The figure shows three views and two pictorial views of one solid part (mm, origin at its lowest corner). Answer the questions. Round coordinates to 2 decimals unless told otherwise and drop trailing zeros. Order: outer loops, then holes, each group sorted by start corner. A loop starts at its lowest first (then second) coordinate and runs counter-clockwise, first axis right, second up. Notation, with made-up numbers: (-4.75, 57) - (1.25, 57) arc R21 ccw to (1.25, 63) - close; hole circle Ø6 at (-28, -29.5). An arc over 180 degrees is marked (long way). Answer as a JSON object with one key per item and string values. Group by question number.
Q1. A cutting plane is placed at A-A on z = 2.25. Determine the outline of the cut face in (x, y).
Q2. A cutting plane is placed at C-C on z = 3.1. Determine the outline of the cut face in (x, y).
Q3. Given pin 1 Ø2 at (x, z) = (3.1, 3.1) entering from +Y, flat-ended and moving along its own axis, determine where the tip first touches the part or whether it passes through.
Q4. A cutting plane is placed at D-D on y = 0.45. Determine the outline of the cut face in (x, z).
Q5. Consider line 1 (Z direction, x = 3.1, y = 0.2); line 2 (X direction, y = 0.55, z = 3.1); line 3 (X direction, y = 0.2, z = 4.25). Determine where each line is inside the solid, lowest interval first.
Q6. A cutting plane is placed at B-B on x = 1.75. Determine the outline of the cut face in (y, z).
Q7. The mould has two halves that part along X. Classify the marked faces 1 and 2: pulls with the +X half, pulls with the -X half, needs draft (parallel to the pull), parting line crosses it, or undercut.
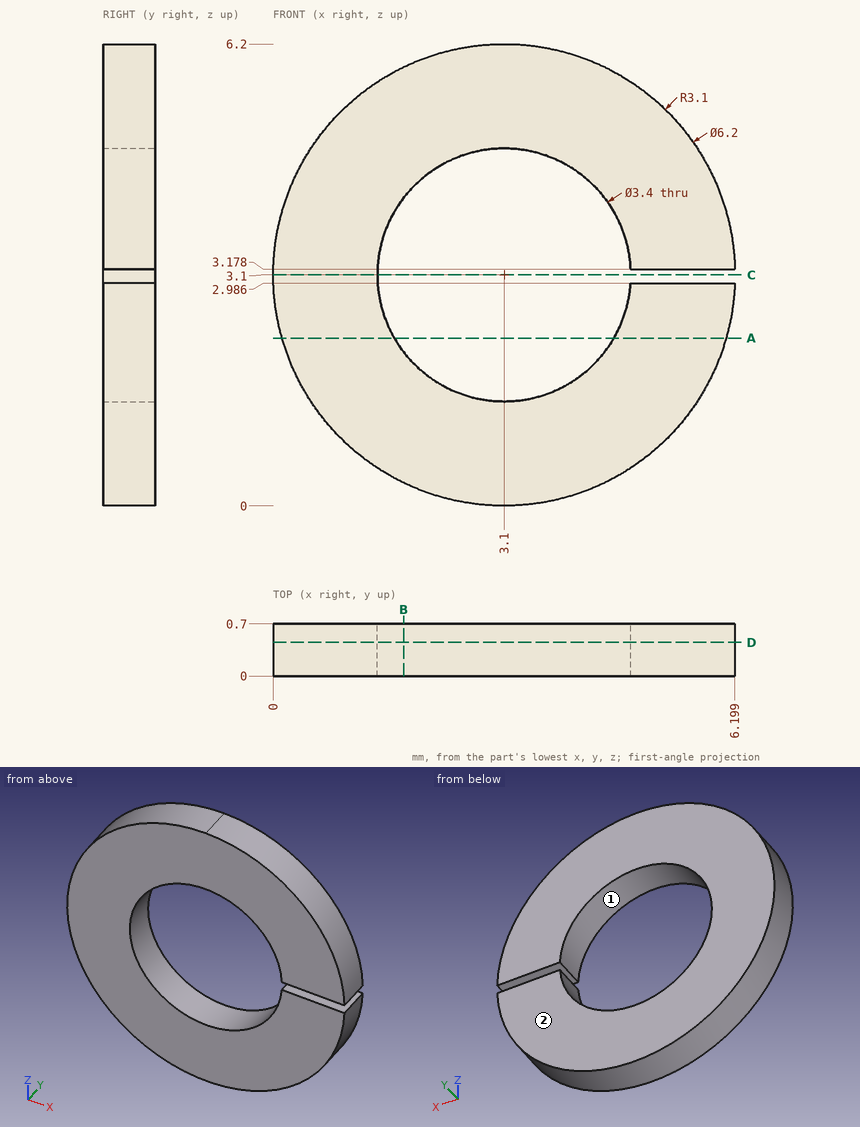
Result set:
{
 "1": {"outline": "(0.12, 0) - (1.63, 0) - (1.63, 0.7) - (0.12, 0.7) - close; (4.57, 0) - (6.08, 0) - (6.08, 0.7) - (4.57, 0.7) - close"},
 "2": {"outline": "(0, 0) - (1.4, 0) - (1.4, 0.7) - (0, 0.7) - close"},
 "3": {"pin 1": "passes through"},
 "4": {"outline": "(4.8, 2.99) arc R1.7 cw (long way) to (4.8, 3.18) - (6.2, 3.18) arc R3.1 ccw (long way) to (6.2, 2.99) - close"},
 "5": {"line 1": "z = 0 to 1.4, 4.8 to 6.2", "line 2": "x = 0 to 1.4", "line 3": "x = 0.22 to 1.85, 4.35 to 5.98"},
 "6": {"outline": "(0, 0.31) - (0.7, 0.31) - (0.7, 2.07) - (0, 2.07) - close; (0, 4.13) - (0.7, 4.13) - (0.7, 5.89) - (0, 5.89) - close"},
 "7": {"face 1": "undercut", "face 2": "needs draft"}
}
